from build123d import *

# Parameters (mm, degrees)
SKETCH1_W            = 410
SKETCH1_H            = 110
BOSS_EXTRUDE1_DEPTH  = 8.5
M4_CLEARANCE_HOLE1_D = 5
M6_CLEARANCE_HOLE1_D = 7
FILLET1_R            = 2.5
CUT_EXTRUDE1_DEPTH   = 8.5
CUT_EXTRUDE2_DEPTH   = 8.5


with BuildPart() as part:
    # Sketch1 → Boss-Extrude1 (new body)
    with BuildSketch(Plane(origin=(0, 0, 0), x_dir=(1, 0, 0), z_dir=(0, 1, 0))):
        Rectangle(SKETCH1_W, SKETCH1_H)
    extrude(amount=BOSS_EXTRUDE1_DEPTH)

    # M4 Clearance Hole1 (through all)
    with Locations(Plane(origin=(0, 8.5, 0), x_dir=(1, 0, 0), z_dir=(0, 1, 0))):
        with Locations((-195, -40), (-195, 40)):
            Hole(M4_CLEARANCE_HOLE1_D / 2)

    # M6 Clearance Hole1 (through all)
    with Locations(Plane(origin=(0, 8.5, 0), x_dir=(1, 0, 0), z_dir=(0, 1, 0))):
        with Locations((19, 34), (19, -34), (-19, -34), (-19, 34)):
            Hole(M6_CLEARANCE_HOLE1_D / 2)

    # Fillet1
    fillet1_edges = [part.edges().sort_by_distance(p)[0] for p in [
        (205, 4.25, 55),
        (-205, 4.25, 55),
        (-205, 4.25, -55),
        (205, 4.25, -55),
    ]]
    fillet(fillet1_edges, radius=FILLET1_R)

    # Sketch6 → Cut-Extrude1 (cut)
    with BuildSketch(Plane(origin=(0, 8.5, 0), x_dir=(1, 0, 0), z_dir=(0, 1, 0))):
        with BuildLine():
            Line((-22.5, 34), (-22.5, 14))
            ThreePointArc((-22.5, 14), (-19, 10.5), (-15.5, 14))
            Line((-15.5, 14), (-15.5, 34))
            Line((-15.5, 34), (-15.5, 44))
            ThreePointArc((-15.5, 44), (-19, 47.5), (-22.5, 44))
            Line((-22.5, 44), (-22.5, 34))
        make_face()
        with BuildLine():
            Line((22.5, 34), (22.5, 14))
            ThreePointArc((22.5, 14), (19, 10.5), (15.5, 14))
            Line((15.5, 14), (15.5, 34))
            Line((15.5, 34), (15.5, 44))
            ThreePointArc((15.5, 44), (19, 47.5), (22.5, 44))
            Line((22.5, 44), (22.5, 34))
        make_face()
        with BuildLine():
            Line((-22.5, -44), (-22.5, -34))
            Line((-22.5, -34), (-22.5, -14))
            ThreePointArc((-22.5, -14), (-19, -10.5), (-15.5, -14))
            Line((-15.5, -14), (-15.5, -34))
            Line((-15.5, -34), (-15.5, -44))
            ThreePointArc((-15.5, -44), (-19, -47.5), (-22.5, -44))
        make_face()
        with BuildLine():
            Line((15.5, -44), (15.5, -34))
            Line((15.5, -34), (15.5, -14))
            ThreePointArc((15.5, -14), (19, -10.5), (22.5, -14))
            Line((22.5, -14), (22.5, -34))
            Line((22.5, -34), (22.5, -44))
            ThreePointArc((22.5, -44), (19, -47.5), (15.5, -44))
        make_face()
    extrude(amount=-CUT_EXTRUDE1_DEPTH, mode=Mode.SUBTRACT)

    # Sketch7 → Cut-Extrude2 (cut)
    with BuildSketch(Plane(origin=(0, 8.5, 0), x_dir=(1, 0, 0), z_dir=(0, 1, 0))):
        with BuildLine():
            Line((-155, 30.8), (-55, 30.8))
            ThreePointArc((-55, 30.8), (-51.7, 27.5), (-55, 24.2))
            Line((-55, 24.2), (-155, 24.2))
            ThreePointArc((-155, 24.2), (-158.3, 27.5), (-155, 30.8))
        make_face()
        with BuildLine():
            Line((-155, -24.2), (-55, -24.2))
            ThreePointArc((-55, -24.2), (-51.7, -27.5), (-55, -30.8))
            Line((-55, -30.8), (-155, -30.8))
            ThreePointArc((-155, -30.8), (-158.3, -27.5), (-155, -24.2))
        make_face()
        with BuildLine():
            Line((55, -24.2), (155, -24.2))
            ThreePointArc((155, -24.2), (158.3, -27.5), (155, -30.8))
            Line((155, -30.8), (55, -30.8))
            ThreePointArc((55, -30.8), (51.7, -27.5), (55, -24.2))
        make_face()
        with BuildLine():
            Line((155, 30.8), (55, 30.8))
            ThreePointArc((55, 30.8), (51.7, 27.5), (55, 24.2))
            Line((55, 24.2), (155, 24.2))
            ThreePointArc((155, 24.2), (158.3, 27.5), (155, 30.8))
        make_face()
    extrude(amount=-CUT_EXTRUDE2_DEPTH, mode=Mode.SUBTRACT)


solid = part.part
Geometry check sheet. Reference: the model listing, model coordinates, mm. A direction names the side the tool comes from. Round coordinates to 2 decimals unless told otherwise and drop trailing zeros. Write each loop counter-clockwise with the first axis right and the second up, starting at its lowest first coordinate (ties: lowest second). Pieces come first, ordered by that corner, then holes. Notation, with made-up numbers: (-11.5, 33) - (36.5, 33) arc R14 cw to (36.5, 51) - close; hole circle Ø7 at (61, 36.25). An arc over 180 degrees is marked (long way). One line per item, written item: value.
1. Cross-section at C-C on y = 2.75. Give the number of separate pieces and of enclosed holes in the cut face, and give its area (3 significant figures).
The answers:
separate pieces: 1
enclosed holes: 10
area: 41,300 mm^2
2. Cross-section at A-A on x = -19. Record the boundary of the cut face in (y, z).
The answers:
outline: (0, -55) - (8.5, -55) - (8.5, -47.5) - (0, -47.5) - close; (0, -10.5) - (8.5, -10.5) - (8.5, 10.5) - (0, 10.5) - close; (0, 47.5) - (8.5, 47.5) - (8.5, 55) - (0, 55) - close
3. Cross-section at B-B on x = -75.5. Record the boundary of the cut face in (y, z), and give its area (3 significant figures).
The answers:
outline: (0, -55) - (8.5, -55) - (8.5, -30.8) - (0, -30.8) - close; (0, -24.2) - (8.5, -24.2) - (8.5, 24.2) - (0, 24.2) - close; (0, 30.8) - (8.5, 30.8) - (8.5, 55) - (0, 55) - close
area: 823 mm^2
4. Set-up check for faces 1 (the face through (-22.5, 4, 29)), 2 (the face through (-205, 4, 1)): record each of +Z, -Z, +X, -X, +Y, -Y from which the full face is reachable in a straight line by a thin tool's end or side.
The answers:
face 1: +Y, -Y
face 2: +Z, -Z, -X, +Y, -Y
5. Scan lines: L1, parallel to Z at x = -195, y = 4.25; L2, parallel to X at y = 1.5, z = 33; L3, parallel to Z at x = -112, y = 2.5. Record each from-to range of solid material in increasing order.
The answers:
L1: z = -55 to -42.5, -37.5 to 37.5, 42.5 to 55
L2: x = -205 to -22.5, -15.5 to 15.5, 22.5 to 205
L3: z = -55 to -30.8, -24.2 to 24.2, 30.8 to 55
6. Mould release check, pull along Z, two halves, no side actions. Record for faces 3 (the face through (-3, 4, -55)), 4 (the face through (-3, 0, -1)), 5 (the face through (-158.3, 4.3, -27.4)): released by +Z, released by -Z, zero draft, split by the parting line, or undercut.
The answers:
face 3: released by -Z
face 4: zero draft
face 5: undercut
